Check sheet for the modelled part. Datum: model origin and axes. Units: mm. Coordinates: 2 decimals unless noted, no trailing zeros. Write each loop counter-clockwise with the first axis right and the second up, starting at its lowest first coordinate (ties: lowest second). Pieces come first, ordered by that corner, then holes. Notation, with made-up numbers: M -7,-19 L 25,-19 A20 cw 25,1 Z; hole C 43.5,62 d3. An arc over 180 degrees is marked long. Answer as CSV lines item,"result". Start each with the question number.
1) Section check B-B (y = 2.25). State how many separate pieces and enclosed holes the cut face has, and give its area (3 significant figures).
2) Section check A-A (x = -20.5). Record the cut outline in (y, z) (3 decimals).
3) Material ranges on L1, parallel to X at y = 2.85, z = -18; L2, parallel to X at y = 0.85, z = 35; L3, parallel to Z at x = 6, y = 1.65, recorded low to high. Write a range as [from, to].
4) Section check D-D (z = -12.5). Record the cut outline in (x, y) (3 decimals).
5) Section check C-C (x = 40.5). Record the cut outline in (y, z) (3 decimals).
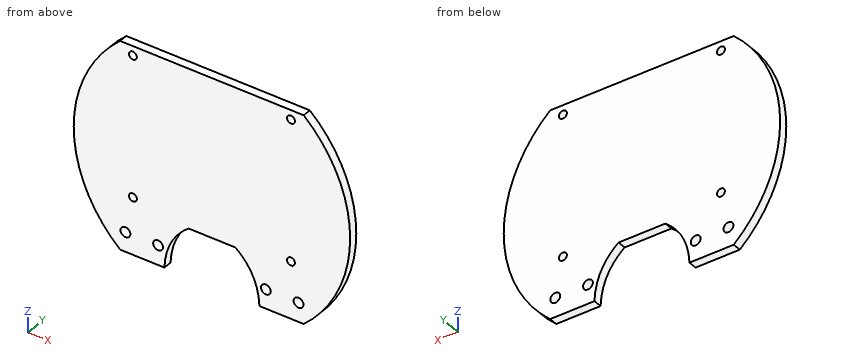
from build123d import *

# Parameters (mm, degrees)
SKETCH1_R           = 50.8
BOSS_EXTRUDE1_DEPTH = 3.175
SKETCH2_W           = 114.887790664
SKETCH2_H           = 17.737062418
CUT_EXTRUDE1_DEPTH  = 3.175
SKETCH6_R           = 1.4605
CUT_EXTRUDE2_DEPTH  = 3.175
SKETCH8_R           = 1.81159506
SKETCH8_R_2         = 1.809329071
SKETCH8_R_3         = 1.797728754
SKETCH8_R_4         = 1.815627059
CUT_EXTRUDE4_DEPTH  = 3.175


with BuildPart() as part:
    # Sketch1 → Boss-Extrude1 (new body)
    with BuildSketch(Plane(origin=(0, 0, 0), x_dir=(1, 0, 0), z_dir=(0, 1, 0))):
        Circle(SKETCH1_R)
    extrude(amount=BOSS_EXTRUDE1_DEPTH)

    # Sketch2 → Cut-Extrude1 (cut)
    with BuildSketch(Plane(origin=(0, 3.175, 0), x_dir=(1, 0, 0), z_dir=(0, 1, 0))):
        with BuildLine():
            Line((-53.141111112, 55.715142418), (61.746679552, 55.715142418))
            Line((61.746679552, 55.715142418), (61.746679552, 37.97808))
            Line((61.746679552, 37.97808), (17.466405486, 37.97808))
            add(Edge.make_bspline(
                [(17.466405486, 37.97808), (17.038082166, 26.714286782), (8.597103322, 20.19808)],
                knots=[0, 0, 0, 1, 1, 1], degree=2))
            Line((8.597103322, 20.19808), (-8.597103322, 20.19808))
            add(Edge.make_bspline(
                [(-17.466405486, 37.97808), (-17.038082166, 26.714286782), (-8.597103322, 20.19808)],
                knots=[0, 0, 0, 1, 1, 1], degree=2))
            Line((-17.466405486, 37.97808), (-53.141111112, 37.97808))
            Line((-53.141111112, 37.97808), (-53.141111112, 55.715142418))
        make_face()
        with Locations((4.30278422, -46.846611209)):
            Rectangle(SKETCH2_W, SKETCH2_H)
    extrude(amount=-CUT_EXTRUDE1_DEPTH, mode=Mode.SUBTRACT)

    # Sketch6 → Cut-Extrude2 (cut)
    with BuildSketch(Plane(origin=(0, 3.175, 0), x_dir=(1, 0, 0), z_dir=(0, 1, 0))):
        with Locations((-29.0576, 17.10182)):
            Circle(SKETCH6_R)
        with Locations((29.0576, 17.10182)):
            Circle(SKETCH6_R)
        with Locations((29.0576, -34.53638)):
            Circle(SKETCH6_R)
        with Locations((-29.0576, -34.53638)):
            Circle(SKETCH6_R)
    extrude(amount=-CUT_EXTRUDE2_DEPTH, mode=Mode.SUBTRACT)

    # Sketch8 → Cut-Extrude4 (cut)
    with BuildSketch(Plane.XZ):
        with Locations((-31.799566939, -30.819765523)):
            Circle(SKETCH8_R)
        with Locations((-19.785366939, -30.819765523)):
            Circle(SKETCH8_R_2)
        with Locations((19.830913185, -30.993944368)):
            Circle(SKETCH8_R_3)
        with Locations((31.845113185, -30.993944368)):
            Circle(SKETCH8_R_4)
    extrude(amount=-CUT_EXTRUDE4_DEPTH, mode=Mode.SUBTRACT)


solid = part.part
Results found:
1,separate pieces,"1"
1,enclosed holes,"8"
1,area,"6,330 mm2"
2,outline,"M 0,-37.978 L 3.175,-37.978 L 3.175,-32.482 L 0,-32.482 Z; M 0,-29.158 L 3.175,-29.158 L 3.175,37.978 L 0,37.978 Z"
3,L1,"x = [-47.5, -30.21], [-27.91, 27.91], [30.21, 47.5]"
3,L2,"x = [-36.82, -30.44], [-27.67, 27.67], [30.44, 36.82]"
3,L3,"z = [-20.2, 37.98]"
4,outline,"M -49.238,0 L 49.238,0 L 49.238,3.175 L -49.238,3.175 Z"
5,outline,"M 0,-30.666 L 3.175,-30.666 L 3.175,30.666 L 0,30.666 Z"
